```python
from build123d import *

# Parameters (mm, degrees)
CROQUIS2_W              = 315
CROQUIS2_H              = 20
SALIENTE_EXTRUIR1_DEPTH = 375
CORTAR_EXTRUIR1_REACH   = 398.622
CROQUIS3_R              = 20


with BuildPart() as part:
    # Croquis2 → Saliente-Extruir1 (new body)
    with BuildSketch(Plane(origin=(0, 0, 360), x_dir=(-1, 0, 0), z_dir=(0, 0, -1))):
        with Locations((7.754092983, 192.834413862)):
            Rectangle(CROQUIS2_W, CROQUIS2_H)
    extrude(amount=SALIENTE_EXTRUIR1_DEPTH)

    # Croquis3 → Cortar-Extruir1 (cut, up to next)
    with BuildSketch(Plane(origin=(0, 202.834413862, 0), x_dir=(1, 0, 0), z_dir=(0, 1, 0)), mode=Mode.PRIVATE) as cortar_extruir1_sk1:
        with Locations(Location((-107.754092983, -25, 0), (0, 0, 270))):
            Circle(CROQUIS3_R)
    cortar_extruir1_tool1 = extrude(cortar_extruir1_sk1.sketch, amount=-CORTAR_EXTRUIR1_REACH, mode=Mode.PRIVATE) & part.part
    # Croquis3 → Cortar-Extruir1 (cut, up to next)
    with BuildSketch(Plane(origin=(0, 202.834413862, 0), x_dir=(1, 0, 0), z_dir=(0, 1, 0)), mode=Mode.PRIVATE) as cortar_extruir1_sk2:
        with Locations(Location((-7.754092983, -25, 0), (0, 0, 270))):
            Circle(CROQUIS3_R)
    cortar_extruir1_tool2 = extrude(cortar_extruir1_sk2.sketch, amount=-CORTAR_EXTRUIR1_REACH, mode=Mode.PRIVATE) & part.part
    # Croquis3 → Cortar-Extruir1 (cut, up to next)
    with BuildSketch(Plane(origin=(0, 202.834413862, 0), x_dir=(1, 0, 0), z_dir=(0, 1, 0)), mode=Mode.PRIVATE) as cortar_extruir1_sk3:
        with Locations(Location((92.245907017, -25, 0), (0, 0, 270))):
            Circle(CROQUIS3_R)
    cortar_extruir1_tool3 = extrude(cortar_extruir1_sk3.sketch, amount=-CORTAR_EXTRUIR1_REACH, mode=Mode.PRIVATE) & part.part
    add(cortar_extruir1_tool1.solids().sort_by_distance((-107.754093, 202.834414, 25))[0], mode=Mode.SUBTRACT)
    add(cortar_extruir1_tool2.solids().sort_by_distance((-7.754093, 202.834414, 25))[0], mode=Mode.SUBTRACT)
    add(cortar_extruir1_tool3.solids().sort_by_distance((92.245907, 202.834414, 25))[0], mode=Mode.SUBTRACT)


solid = part.part
```
CAD build for the part. Positions are in the model's coordinates, mm. Round coordinates to 2 decimals unless told otherwise and drop trailing zeros. Write each loop counter-clockwise with the first axis right and the second up, starting at its lowest first coordinate (ties: lowest second). Pieces come first, ordered by that corner, then holes.
Item 1: Band-saw the part on C-C on y = 186.5. Write the cut outline in (x, z).
Filled in:
outline: (-165.25, -15) - (149.75, -15) - (149.75, 360) - (-165.25, 360) - close; hole circle Ø40 at (-107.75, 25); hole circle Ø40 at (-7.75, 25); hole circle Ø40 at (92.25, 25)
Item 2: Band-saw the part on D-D on x = -119. Write the cut outline in (y, z), then the cut area to 3 significant figures.
Filled in:
outline: (182.83, -15) - (202.83, -15) - (202.83, 8.46) - (182.83, 8.46) - close; (182.83, 41.54) - (202.83, 41.54) - (202.83, 360) - (182.83, 360) - close
area: 6,840 mm2
Item 3: Band-saw the part on A-A on z = 25. Write the cut outline in (x, y), then the cut area to 3 significant figures.
Filled in:
outline: (-165.25, 182.83) - (-127.75, 182.83) - (-127.75, 202.83) - (-165.25, 202.83) - close; (-87.75, 182.83) - (-27.75, 182.83) - (-27.75, 202.83) - (-87.75, 202.83) - close; (12.25, 182.83) - (72.25, 182.83) - (72.25, 202.83) - (12.25, 202.83) - close; (112.25, 182.83) - (149.75, 182.83) - (149.75, 202.83) - (112.25, 202.83) - close
area: 3,900 mm2
Item 4: Mould opens along X. For faces 1 (the cylindrical face through (-101.747, 192.974, 44.076)), 2 (the flat face through (-6, 182.834, 175)), 3 (the flat face through (-165.254, 193, 175)) say: released by +X, released by -X, zero draft, split by the parting line, or undercut.
Filled in:
face 1: undercut
face 2: zero draft
face 3: released by -X
Item 5: Band-saw the part on B-B on x = 86. Write the cut outline in (y, z).
Filled in:
outline: (182.83, -15) - (202.83, -15) - (202.83, 6) - (182.83, 6) - close; (182.83, 44) - (202.83, 44) - (202.83, 360) - (182.83, 360) - close
Item 6: Drill centre lines: L1, parallel to X at y = 189, z = 25; L2, parallel to X at y = 199.25, z = 40; L3, parallel to Z at x = -122.5, y = 191. Where is each one in solid material? Low to high.
Filled in:
L1: x = -165.25 to -127.75, -87.75 to -27.75, 12.25 to 72.25, 112.25 to 149.75
L2: x = -165.25 to -120.98, -94.53 to -20.98, 5.47 to 79.02, 105.47 to 149.75
L3: z = -15 to 11.49, 38.51 to 360
